from build123d import *

# Parameters (mm, degrees)
F2_R = 2.54
F3_R = 1.27


with BuildPart() as f1:
    # F0 (on Front) → F1 (revolve)
    with BuildSketch(Plane.XZ):
        Polygon((5.08, 0), (8.255, 0), (5.08, 5.499261), (7.62, 5.499261), (4.445, 10.998523), (6.985, 10.998523), (3.81, 16.497784), (6.35, 16.497784), (3.81, 20.897193), (0, 20.897193), (0, 8.798818), align=None)
    revolve(axis=Axis((0, 0, 14.848006), (0, 0, -1)))

    # F2
    f2_edges = [f1.edges().sort_by_distance(p)[0] for p in [
        (-5.08, 0, 0),
    ]]
    fillet(f2_edges, radius=F2_R)

    # F3
    f3_edges = [f1.edges().sort_by_distance(p)[0] for p in [
        (-5.08, 0, 5.499261),
        (-4.445, 0, 10.998523),
        (-3.81, 0, 16.497784),
    ]]
    fillet(f3_edges, radius=F3_R)


solid = f1.part
Read the model definition and answer for the solid it produces. Units are mm, in the model's axes. A direction names the side the tool comes from. Round coordinates to 2 decimals unless told otherwise and drop trailing zeros. Order: outer loops, then holes, each group sorted by start corner. A loop starts at its lowest first (then second) coordinate and runs counter-clockwise, first axis right, second up.
1) The mould has two halves that part along Y. Classify faces 3 (the face through (6, -4, 0)), 4 (the face through (-0.735, -5.598, 8.919)), 5 (the face through (-1.366, 1.047, 5.818)): released by +Y, released by -Y, zero draft, split by the parting line, or undercut.
2) Straight lines are drawn through the part: L1, parallel to Z at x = -0.75, y = -5.5; L2, parallel to Z at x = -5.75, y = 1.25; L3, parallel to Y at x = -2.5, z = 3.75. For each, find the intervals that lie inside material, in ascending order.
3) Flat-ended cylindrical pins translate along their axes: pin 1 (6.5 mm diameter, centred on x = 1.5, y = 0.5, fed in from -Z); pin 2 (1 mm diameter, centred on x = -5.5, z = 17, fed in from -Y); pin 3 (5 mm diameter, centred on y = -2.5, z = 6, fed in from +X). Find the tip coordinate at first contact, or state that the pin passes through.
4) For faces 1 (the face through (4.779, -1.505, 14.418)), 2 (the face through (-3.121, 2.393, 20.684)), determine the directions among +Z, -Z, +X, -X, +Y, -Y from which every point of the face is accessible in a straight line to the end or side of a thin tool.
5) The part is cut by section A-A on z = 4. Write down the section's boundary in (x, y).
Resolved:
1. face 3: zero draft
1. face 4: split by the parting line
1. face 5: undercut
2. L1: z = 0.2 to 9.08, 10.37 to 13.48, 16.41 to 17.88
2. L2: z = 0.09 to 8.51, 10.75 to 12.9, 16.49 to 17.3
2. L3: y = -5.57 to -1.5, 1.5 to 5.57
3. pin 1: stops at z = 0.67
3. pin 2: stops at y = -3.58
3. pin 3: stops at x = 7.62
4. face 1: none
4. face 2: +Z
5. outline: circle Ø12.06 at (0, 0); hole circle Ø5.54 at (0, 0)
